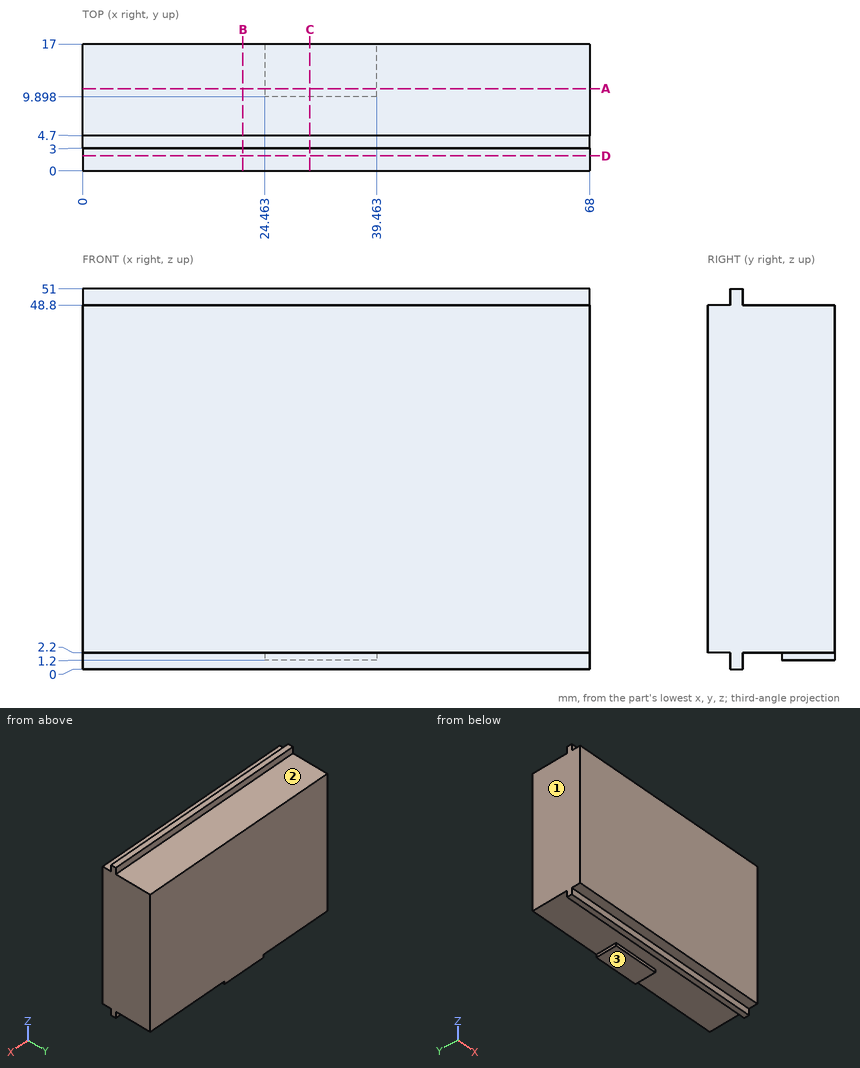
Design review of the part shown in the three views and the two pictorial views. Dimensions are in mm from the part's minimum x, y and z. A direction names the side the tool comes from. Coordinates: 2 decimals unless noted, no trailing zeros. Write each loop counter-clockwise with the first axis right and the second up, starting at its lowest first coordinate (ties: lowest second). Pieces come first, ordered by that corner, then holes.
(1) Add section A-A on y = 11. Give the boundary of the cut face in (x, z), then the cut area to 3 significant figures.
(2) Tool access review of the marked faces 1, 2 and 3: name each direction out of +Z, -Z, +X, -X, +Y, -Y from which nothing blocks a thin tool from reaching the whole face with its end or side.
(3) Add section D-D on y = 2. Give the boundary of the cut face in (x, z).
(4) Add section B-B on x = 21.5. Give the boundary of the cut face in (y, z), then the cut area to 3 significant figures.
(5) Add section C-C on x = 30.5. Give the boundary of the cut face in (y, z), then the cut area to 3 significant figures.
(6) Wall thickness on probe 1 along Y at (x, z) = (43, 2); probe 2 along Z at (x, y) = (13, 14.75): over which ranges is each line inside the solid? List them lowest first.
(7) For pin 1 Ø0.8 at (x, z) = (34.5, 2) entering from -Y; pin 2 Ø1.1 at (x, z) = (18, 50) entering from -Y; pin 3 Ø8 at (x, y) = (32.5, 14.5) entering from -Z; pin 4 Ø3.5 at (x, y) = (21, 13) entering from +Z, all flat-tipped, find the tip position at first contact; note any pin that passes through.
Answer sheet:
1. outline: (0, 2.2) - (24.46, 2.2) - (24.46, 1.2) - (39.46, 1.2) - (39.46, 2.2) - (68, 2.2) - (68, 48.8) - (0, 48.8) - close
1. area: 3,180 mm2
2. face 1: +Z, -Z, -X, +Y, -Y
2. face 2: +Z, +X, -X, +Y
2. face 3: -Z, +X, -X, +Y
3. outline: (0, 2.2) - (68, 2.2) - (68, 48.8) - (0, 48.8) - close
4. outline: (0, 2.2) - (3, 2.2) - (3, 0) - (4.7, 0) - (4.7, 2.2) - (17, 2.2) - (17, 48.8) - (4.7, 48.8) - (4.7, 51) - (3, 51) - (3, 48.8) - (0, 48.8) - close
4. area: 800 mm2
5. outline: (0, 2.2) - (3, 2.2) - (3, 0) - (4.7, 0) - (4.7, 2.2) - (9.9, 2.2) - (9.9, 1.2) - (17, 1.2) - (17, 48.8) - (4.7, 48.8) - (4.7, 51) - (3, 51) - (3, 48.8) - (0, 48.8) - close
5. area: 807 mm2
6. probe 1: y = 3 to 4.7
6. probe 2: z = 2.2 to 48.8
7. pin 1: stops at y = 0
7. pin 2: stops at y = 3
7. pin 3: stops at z = 1.2
7. pin 4: stops at z = 48.8
